Geometry check sheet. Reference: the model listing, model coordinates, mm. Face numbers are marked on the shaded views. A direction names the side the tool comes from. Coordinates: 2 decimals unless noted, no trailing zeros. Loops run counter-clockwise (first coordinate to the right, second up) from the corner with the lowest first, then second, coordinate; pieces in that order, holes last. Notation, with made-up numbers: M 67.5,-5.5 L 121.5,-5.5 A25 ccw 121.5,10.5 Z; hole C -13.5,54 d8. An arc over 180 degrees is marked long. Use CSV: the item, a comma, the result in double quotes.
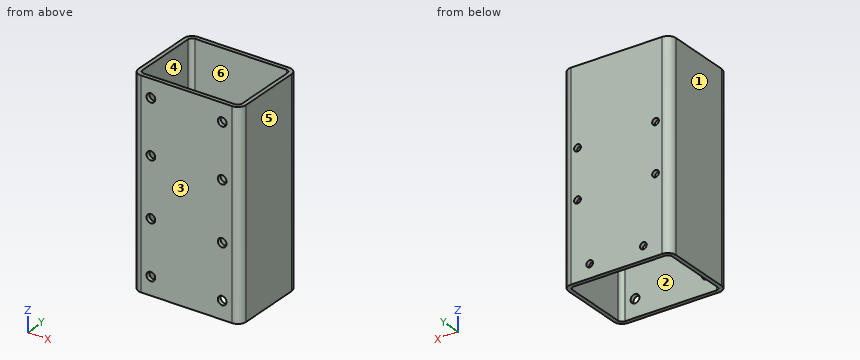
```python
from build123d import *

# Parameters (mm, degrees)
BOSS_EXTRUDE1_DEPTH             = 75
BOSS_EXTRUDE1_DEPTH_BACK        = 75
F_6_5_6_5_DIAMETER_HOLE1_D      = 6.5
F_6_5_6_5_DIAMETER_HOLE1_DEPTH  = 3
TAP_DRILL_FOR_M6X1_0_TAP1_D     = 5
TAP_DRILL_FOR_M6X1_0_TAP1_DEPTH = 3


with BuildPart() as part:
    # Sketch1 → Boss-Extrude1 (new, two sides: drawn at the far end of the back side and taken through both)
    with BuildSketch(Plane.XY.offset(-BOSS_EXTRUDE1_DEPTH_BACK)):
        with BuildLine():
            Line((-34, -30), (34, -30))
            ThreePointArc((34, -30), (38.242640687, -28.242640687), (40, -24))
            Line((40, -24), (40, 24))
            ThreePointArc((40, 24), (38.242640687, 28.242640687), (34, 30))
            Line((34, 30), (-34, 30))
            ThreePointArc((-34, 30), (-38.242640687, 28.242640687), (-40, 24))
            Line((-40, 24), (-40, -24))
            ThreePointArc((-40, -24), (-38.242640687, -28.242640687), (-34, -30))
        make_face()
        with BuildLine():
            Line((-34, 27), (34, 27))
            ThreePointArc((34, 27), (36.121320344, 26.121320344), (37, 24))
            Line((37, 24), (37, -24))
            ThreePointArc((37, -24), (36.121320344, -26.121320344), (34, -27))
            Line((34, -27), (-34, -27))
            ThreePointArc((-34, -27), (-36.121320344, -26.121320344), (-37, -24))
            Line((-37, -24), (-37, 24))
            ThreePointArc((-37, 24), (-36.121320344, 26.121320344), (-34, 27))
        make_face(mode=Mode.SUBTRACT)
    extrude(amount=BOSS_EXTRUDE1_DEPTH + BOSS_EXTRUDE1_DEPTH_BACK)

    # Ø6.5 (6.5) Diameter Hole1
    with Locations(Plane(origin=(-26.5, -30, 61.75), x_dir=(0, 0, -1), z_dir=(0, -1, 0))):
        with Locations((0, 0), (0, 53), (40, 53), (40, 0), (83.5, 0), (83.5, 53), (123.5, 53), (123.5, 0)):
            Hole(F_6_5_6_5_DIAMETER_HOLE1_D / 2, depth=F_6_5_6_5_DIAMETER_HOLE1_DEPTH)

    # Tap Drill for M6x1.0 Tap1
    with Locations(Plane(origin=(29.000000001, 30, -18), x_dir=(1, 0, 0), z_dir=(0, 1, 0))):
        with Locations((0, 0), (0, -36), (-58, -36), (-58, 0), (-49, 47), (-9, 47)):
            Hole(TAP_DRILL_FOR_M6X1_0_TAP1_D / 2, depth=TAP_DRILL_FOR_M6X1_0_TAP1_DEPTH)


solid = part.part
```
1. Gauge pin test, flat ends, axial feed: P1, Ø4.5, axis at x = -29, z = 18, coming from the +Y side; P2, Ø4, axis at x = 26.5, z = 21.75, coming from the -Y side. Record the tip position at first contact, or that the pin passes through.
The answers:
P1,"y = -27"
P2,"y = 27"
2. Set-up check for the marked faces 5 and 6: record each of +Z, -Z, +X, -X, +Y, -Y from which the full face is reachable in a straight line by a thin tool's end or side.
The answers:
face 5,"+Z, -Z, +X, +Y, -Y"
face 6,"+Z, -Z"
3. Section check A-A, the plane y = -6.5. Record the cut outline in (x, z).
The answers:
outline,"M -40,-75 L -37,-75 L -37,75 L -40,75 Z; M 37,-75 L 40,-75 L 40,75 L 37,75 Z"
4. Section check C-C, the plane z = 4. Record the cut outline in (x, y).
The answers:
outline,"M -40,-24 A6 ccw -34,-30 L 34,-30 A6 ccw 40,-24 L 40,24 A6 ccw 34,30 L -34,30 A6 ccw -40,24 Z; hole M -37,-24 A3 ccw -34,-27 L 34,-27 A3 ccw 37,-24 L 37,24 A3 ccw 34,27 L -34,27 A3 ccw -37,24 Z"
5. Release check for a two-part mould opening along Y. For the marked faces 1, 2, 3 and 4 record: +Y half, -Y half, draft (parallel to the pull), parting line (faces both ways), or undercut.
The answers:
face 1,"draft"
face 2,"undercut"
face 3,"-Y half"
face 4,"undercut"
6. Section check B-B, the plane z = 61.75. Record the cut outline in (x, y), plus the area to 3 significant figures.
The answers:
outline,"M -40,-24 A6 ccw -34,-30 L -29.75,-30 L -29.75,-27 L -34,-27 A3 cw -37,-24 L -37,24 A3 cw -34,27 L 34,27 A3 cw 37,24 L 37,-24 A3 cw 34,-27 L 29.75,-27 L 29.75,-30 L 34,-30 A6 ccw 40,-24 L 40,24 A6 ccw 34,30 L -34,30 A6 ccw -40,24 Z; M -23.25,-30 L 23.25,-30 L 23.25,-27 L -23.25,-27 Z"
area,"742 mm^2"
7. Thickness scan on line 1 (Z direction, x = -29, y = 27.7); line 2 (Y direction, x = -11, z = -15.5); line 3 (X direction, y = -7, z = -11). Record the ranges inside material, lowest first. Write a range as [from, to].
The answers:
line 1,"[-75, -20.5], [-15.5, 15.5], [20.5, 75]"
line 2,"[-30, -27], [27, 30]"
line 3,"[-40, -37], [37, 40]"
